from build123d import *

# Parameters (mm, degrees)
ESQUISSE1_W             = 361.95
ESQUISSE1_H             = 601.98
BOSS_EXTRU_1_DEPTH      = 130.175
ESQUISSE3_W             = 355.6
ESQUISSE3_H             = 127
ENL_V_MAT_EXTRU_2_DEPTH = 3.175
ESQUISSE4_W             = 355.6
ESQUISSE4_H             = 595.63
ENL_V_MAT_EXTRU_3_DEPTH = 127
ESQUISSE5_W             = 355.6
ESQUISSE5_H             = 127
ENL_V_MAT_EXTRU_4_DEPTH = 3.175


with BuildPart() as part:
    # Esquisse1 → Boss.-Extru.1 (new, symmetric)
    with BuildSketch(Plane.XY):
        Rectangle(ESQUISSE1_W, ESQUISSE1_H)
    extrude(amount=BOSS_EXTRU_1_DEPTH, both=True)

    # Esquisse3 → Enlèv. mat.-Extru.2 (cut)
    with BuildSketch(Plane.XY.offset(130.175)):
        with Locations((0, -234.315)):
            Rectangle(ESQUISSE3_W, ESQUISSE3_H)
    extrude(amount=-ENL_V_MAT_EXTRU_2_DEPTH, mode=Mode.SUBTRACT)

    # Esquisse4 → Enlèv. mat.-Extru.3 (cut, symmetric)
    with BuildSketch(Plane.XY):
        Rectangle(ESQUISSE4_W, ESQUISSE4_H)
    extrude(amount=ENL_V_MAT_EXTRU_3_DEPTH, both=True, mode=Mode.SUBTRACT)

    # Esquisse5 → Enlèv. mat.-Extru.4 (cut)
    with BuildSketch(Plane(origin=(0, 0, -130.175), x_dir=(-1, 0, 0), z_dir=(0, 0, -1))):
        with Locations((0, 234.315)):
            Rectangle(ESQUISSE5_W, ESQUISSE5_H)
    extrude(amount=-ENL_V_MAT_EXTRU_4_DEPTH, mode=Mode.SUBTRACT)


solid = part.part
For this review, take the finished solid that the model builds, in its own axes (mm). A direction names the side the tool comes from. Coordinates: 2 decimals unless noted, no trailing zeros. Order: outer loops, then holes, each group sorted by start corner. A loop starts at its lowest first (then second) coordinate and runs counter-clockwise, first axis right, second up. Notation, with made-up numbers: (-35.75, 50.5) - (-20.75, 50.5) arc R21 ccw to (-20.75, 73.5) - close; hole circle Ø3 at (-1.5, 18.25). An arc over 180 degrees is marked (long way). Answer as CSV lines item,"result". Start each with the question number.
1) Draft analysis for pull direction Y (two halves, no side actions). For faces 6 (the flat face through (-177.8, -4, -2)), 7 (the flat face through (-3, 71, 130.175)), 8 (the flat face through (-3, -300.99, 2)), state which applies: +Y half, -Y half, draft (parallel to the pull), parting line (faces both ways), or undercut.
2) To check wall thickness, follow line 1 along Z through (x, y) = (-145, 139) (3 decimals); line 2 along X through (y, z) = (109.5, 34.5) (3 decimals); line 3 along Y through (x, z) = (58, 5.5) (3 decimals). State the ranges of each line that lie inside material, in increasing order. Write a range as [from, to].
3) Machinability: for faces 1 (the flat face through (-2, -60, -127)), 2 (the flat face through (-180.975, -4, 2)), 3 (the flat face through (2, 297.815, -3)), 4 (the flat face through (-2, -297.815, 3)), 5 (the flat face through (180.975, -4, 2)), which of the approach directions +Z, -Z, +X, -X, +Y, -Y give a long, thin tool a straight path to every point of the face, cutting with its end or side? Answer none if there is none.
4) Add section C-C (y = 10). State the section outline as (x, z) points (3 decimals), then the cut area to 3 significant figures.
5) Add section A-A (x = -20). State the section outline as (y, z) points (3 decimals), then the cut area to 3 significant figures.
6) Add section B-B (z = 58). State the section outline as (x, y) points (3 decimals), then the cut area to 3 significant figures.
7) Add section D-D (y = 223.5). State the section outline as (x, z) points (3 decimals), then the cut area to 3 significant figures.
8) Insertion check: P1, Ø3, axis at x = -120.5, y = -203.5, coming from the +Z side; P2, Ø5, axis at x = 37.5, y = 239, coming from the -Z side. Each pin has a flat end and moves straight along its axis. Give the tip position at first contact, or say it passes through.
Result:
1,face 6,"undercut"
1,face 7,"draft"
1,face 8,"-Y half"
2,line 1,"[-130.175, -127], [127, 130.175]"
2,line 2,"[-180.975, -177.8], [177.8, 180.975]"
2,line 3,"[-300.99, -297.815], [297.815, 300.99]"
3,face 1,"none"
3,face 2,"+Z, -Z, -X, +Y, -Y"
3,face 3,"-Z"
3,face 4,"+Z"
3,face 5,"+Z, -Z, +X, +Y, -Y"
4,outline,"(-180.975, -130.175) - (180.975, -130.175) - (180.975, 130.175) - (-180.975, 130.175) - close; hole (-177.8, -127) - (177.8, -127) - (177.8, 127) - (-177.8, 127) - close"
4,area,"3,910 mm^2"
5,outline,"(-300.99, -130.175) - (170.815, -130.175) - (170.815, -127) - (-297.815, -127) - (-297.815, 130.175) - (-300.99, 130.175) - close; (-170.815, 127) - (297.815, 127) - (297.815, -130.175) - (300.99, -130.175) - (300.99, 130.175) - (-170.815, 130.175) - close"
5,area,"4,630 mm^2"
6,outline,"(-180.975, -300.99) - (180.975, -300.99) - (180.975, 300.99) - (-180.975, 300.99) - close; hole (-177.8, -297.815) - (177.8, -297.815) - (177.8, 297.815) - (-177.8, 297.815) - close"
6,area,"6,080 mm^2"
7,outline,"(-180.975, -130.175) - (-177.8, -130.175) - (-177.8, 127) - (177.8, 127) - (177.8, -130.175) - (180.975, -130.175) - (180.975, 130.175) - (-180.975, 130.175) - close"
7,area,"2,780 mm^2"
8,P1,"z = -127"
8,P2,"z = 127"
